Geometry: see drawing. Coordinates: mm, zero at the bounding-box minimum. A direction names the side the tool comes from. Round coordinates to 2 decimals unless told otherwise and drop trailing zeros. Loops run counter-clockwise (first coordinate to the right, second up) from the corner with the lowest first, then second, coordinate; pieces in that order, holes last. Notation, with made-up numbers: M 72,-31 L 82,-31 A26 cw 82,3 Z; hole C 68.25,46.5 d3. An arc over 180 degrees is marked long. Answer as a JSON object with one key per item and string values.
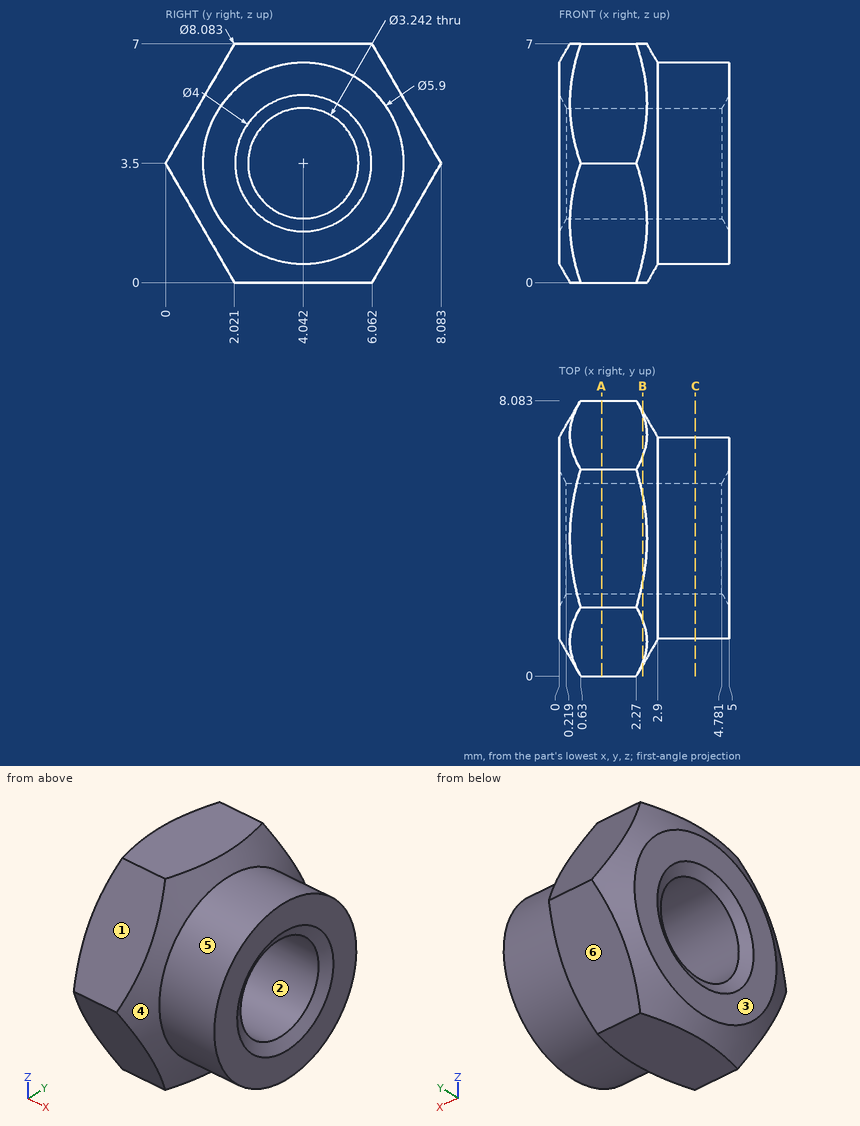
1) Section query B-B (x = 2.45). Return the cut outline in (y, z) (1 decimal).
Results:
{"outline": "M 0.4,2.9 L 1.7,0.6 A3.7 ccw 2.8,0 L 5.3,0 A3.7 ccw 6.4,0.6 L 7.7,2.9 A3.7 ccw 7.7,4.1 L 6.4,6.4 A3.7 ccw 5.3,7 L 2.8,7 A3.7 ccw 1.7,6.4 L 0.4,4.1 A3.7 ccw Z; hole C 4,3.5 d3.2"}
2) Ray query, line 1 (Y direction, x = 3.05, z = 3.5); line 2 (Z direction, x = 0.9, y = 4); line 3 (Y direction, x = 0.35, z = 4) (1 decimal). Return the intervals inside material, ascending.
Results:
{"line 1": "1.09 to 2.42, 5.66 to 6.99", "line 2": "0 to 1.88, 5.12 to 7", "line 3": "0.5 to 2.5, 5.6 to 7.6"}
3) Section query C-C (x = 4). Return the cut outline in (y, z), and give its area (3 significant figures).
Results:
{"outline": "C 4.04,3.5 d5.9; hole C 4.04,3.5 d3.24", "area": "19.1 mm2"}
4) Reachability of the marked faces 5 and 6 from +Z, -Z, +X, -X, +Y, -Y: full face, straight path, thin tool, end or side. Return the list, or none.
Results:
{"face 5": "+X", "face 6": "-Z, +X, -X, +Y"}
5) Pin query (flat end, axial travel): P1, Ø1.5, axis at x = 1.5, z = 2, coming from the +Y side; P2, Ø1, axis at x = 4.5, z = 3, coming from the +Y side; P3, Ø1, axis at y = 1, z = 4, coming from the -X side; P4, Ø1.5, axis at x = 0.5, z = 4.5, coming from the -Y side (1 decimal). Return the tip coordinate at first contact, or that it passes through.
Results:
{"P1": "y = 7.65", "P2": "y = 6.99", "P3": "x = 0", "P4": "y = 0.1"}
6) Pull-direction query (Y, two-part tool) for the marked faces 1, 2, 3 and 4; classes: +Y half, -Y half, draft (parallel to the pull), parting line (faces both ways), or undercut.
Results:
{"face 1": "-Y half", "face 2": "undercut", "face 3": "draft", "face 4": "parting line"}
7) Section query A-A (x = 1.25). Return the cut outline in (y, z).
Results:
{"outline": "M 0,3.5 L 2.02,0 L 6.06,0 L 8.08,3.5 L 6.06,7 L 2.02,7 Z; hole C 4.04,3.5 d3.24"}
